Source: CAD feature listing. Evaluate the final solid. Frame: model axes, mm. Give positions to 0.01 mm unless a question says otherwise; leave off trailing zeros. Order: outer loops, then holes, each group sorted by start corner. A loop starts at its lowest first (then second) coordinate and runs counter-clockwise, first axis right, second up.
```python
from build123d import *

# Parameters (mm, degrees)
SKETCH_1_W                   = 700
SKETCH_1_H                   = 600
EXTRUDE_1_DEPTH              = 15
SKETCH_2_W                   = 92
SKETCH_2_H                   = 95
CUT_EXTRUDE_1_DEPTH          = 16
HOLE_WIZARD_5_0_5_1_D        = 5
HOLE_WIZARD_6_8_6_8_1_D      = 6.8
HOLE_WIZARD_6_8_6_8_1_DEPTH  = 15
HOLE_WIZARD_M8_1_D           = 9
HOLE_WIZARD_M8_1_DEPTH       = 15
HOLE_WIZARD_M8_1_CBORE_D     = 15
HOLE_WIZARD_M8_1_CBORE_DEPTH = 9
HOLE_WIZARD_4_2_4_2_1_D      = 4.2
HOLE_WIZARD_4_2_4_2_1_DEPTH  = 12.4
HOLE_WIZARD_4_2_4_2_1_TIP    = 1.2618073
HOLE_WIZARD_M80_1_D          = 90
HOLE_WIZARD_M80_1_DEPTH      = 15
HOLE_WIZARD_M39_1_D          = 45
CHAMFER_1_SIZE               = 0.025


with BuildPart() as part:
    # 草图1 → 凸台-拉伸1 (new body)
    with BuildSketch(Plane(origin=(0, 0, -190), x_dir=(-1, 0, 0), z_dir=(0, 0, -1))):
        with Locations((0, 1520)):
            Rectangle(SKETCH_1_W, SKETCH_1_H)
    extrude(amount=-EXTRUDE_1_DEPTH)

    # 草图2 → 切除-拉伸1 (cut, through all)
    with BuildSketch(Plane.XY.offset(-175)):
        with Locations((0, 1267.5)):
            Rectangle(SKETCH_2_W, SKETCH_2_H)
    extrude(amount=-CUT_EXTRUDE_1_DEPTH, mode=Mode.SUBTRACT)

    # Ø5.0 (5) 直径孔1 (through all)
    with Locations(Plane.XY.offset(-175)):
        with Locations((-40.658639918, 1699.341360082), (40.658639918, 1699.341360082), (40.658639918, 1780.658639918), (-40.658639918, 1780.658639918)):
            Hole(HOLE_WIZARD_5_0_5_1_D / 2)

    # Ø6.8 (6.8) 直径孔1
    with Locations(Plane.XY.offset(-175)):
        with Locations((60, 1319.472182943), (60, 1269.472182943), (-60, 1269.472182943), (-60, 1319.472182943), (22.5, 1345), (-22.5, 1345)):
            Hole(HOLE_WIZARD_6_8_6_8_1_D / 2, depth=HOLE_WIZARD_6_8_6_8_1_DEPTH)

    # M8 六角头螺栓的柱形沉头孔1
    with Locations(Plane(origin=(0, 0, -190), x_dir=(-1, 0, 0), z_dir=(0, 0, -1))):
        with Locations((240, 1250), (240, 1430), (240, 1610), (240, 1790), (-240, 1250), (-240, 1430), (-240, 1610), (-240, 1790)):
            CounterBoreHole(HOLE_WIZARD_M8_1_D / 2, HOLE_WIZARD_M8_1_CBORE_D / 2, HOLE_WIZARD_M8_1_CBORE_DEPTH, depth=HOLE_WIZARD_M8_1_DEPTH)

    # Ø4.2 (4.2) 直径孔1
    with Locations(Plane.XY.offset(-175)):
        with Locations((305, 1715), (305, 1755)):
            Hole(HOLE_WIZARD_4_2_4_2_1_D / 2, depth=HOLE_WIZARD_4_2_4_2_1_DEPTH)
            with Locations((0, 0, -(HOLE_WIZARD_4_2_4_2_1_DEPTH + HOLE_WIZARD_4_2_4_2_1_TIP / 2))):  # 118° drill point
                Cone(0, HOLE_WIZARD_4_2_4_2_1_D / 2, HOLE_WIZARD_4_2_4_2_1_TIP, mode=Mode.SUBTRACT)

    # M80 间隙孔1
    with Locations(Plane(origin=(0, 0, -190), x_dir=(-1, 0, 0), z_dir=(0, 0, -1))):
        with Locations((0, 1740)):
            Hole(HOLE_WIZARD_M80_1_D / 2, depth=HOLE_WIZARD_M80_1_DEPTH)

    # M39 间隙孔1 (through all)
    with Locations(Plane.XY.offset(-175)):
        with Locations((-320, 1680), (320, 1680)):
            Hole(HOLE_WIZARD_M39_1_D / 2)

    # 倒角1
    chamfer_1_edges = [part.edges().sort_by_distance(p)[0] for p in [
        (342.5, 1680, -175),
        (-297.5, 1680, -175),
    ]]
    chamfer(chamfer_1_edges, length=CHAMFER_1_SIZE)


solid = part.part
```
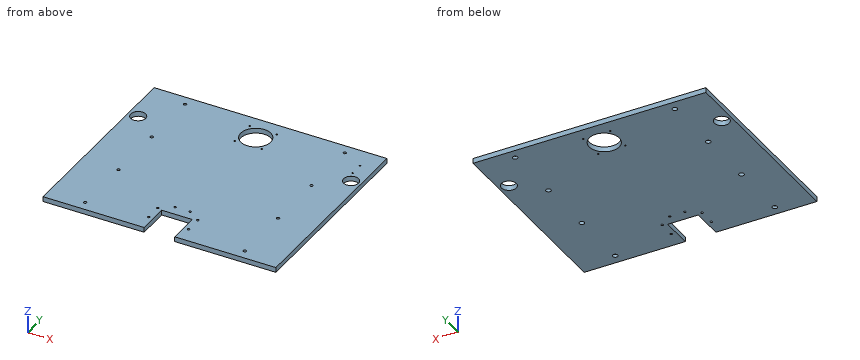
1) Material intervals for L1, parallel to Y at x = -240, z = -182.75; L2, parallel to Y at x = 60, z = -187; L3, parallel to X at y = 1345, z = -180.75, sorted ascending.
Report:
L1: y = 1220 to 1242.5, 1257.5 to 1422.5, 1437.5 to 1602.5, 1617.5 to 1782.5, 1797.5 to 1820
L2: y = 1220 to 1266.07, 1272.87 to 1316.07, 1322.87 to 1820
L3: x = -350 to -25.9, -19.1 to 19.1, 25.9 to 350
2) Pin query (flat end, axial travel): pin 1 (14.5 mm diameter, centred on x = -240, y = 1250, fed in from -Z); pin 2 (6 mm diameter, centred on x = -60, y = 1319.47, fed in from -Z) (3 decimals); pin 3 (2 mm diameter, centred on x = -39, z = -183, fed in from -Y). Return the tip coordinate at first contact, or that it passes through.
Report:
pin 1: stops at z = -181
pin 2: passes through
pin 3: stops at y = 1315
3) Section query B-B, the plane y = 1740. Return the cut outline in (x, z).
Report:
outline: (-350, -190) - (-45, -190) - (-45, -175) - (-350, -175) - close; (45, -190) - (350, -190) - (350, -175) - (45, -175) - close
4) Section query A-A, the plane x = 320. Return the cut outline in (y, z) (3 decimals).
Report:
outline: (1220, -190) - (1657.5, -190) - (1657.5, -175.025) - (1657.475, -175) - (1220, -175) - close; (1702.5, -190) - (1820, -190) - (1820, -175) - (1702.525, -175) - (1702.5, -175.025) - close
